from build123d import *

# Parameters (mm, degrees)
SKETCH1_W                                           = 162
SKETCH1_H                                           = 180
SKETCH1_W_2                                         = 50
SKETCH1_H_2                                         = 4
SKETCH1_W_3                                         = 4
SKETCH1_H_3                                         = 50
BOSS_EXTRUDE2_DEPTH                                 = 4
CUT_EXTRUDE1_REACH                                  = 136.376
SKETCH2_W                                           = 50
SKETCH2_H                                           = 4
CSK_FOR_M3_COUNTERSUNK_FLAT_HEAD_SCREW1_D           = 3.4
CSK_FOR_M3_COUNTERSUNK_FLAT_HEAD_SCREW1_CSINK_D     = 6.3
CSK_FOR_M3_COUNTERSUNK_FLAT_HEAD_SCREW1_CSINK_ANGLE = 90
CSK_FOR_M4_COUNTERSUNK_FLAT_HEAD_SCR_2_COUNT        = 2
CSK_FOR_M4_COUNTERSUNK_FLAT_HEAD_SCR_2_PITCH        = 142
CSK_FOR_M4_COUNTERSUNK_FLAT_HEAD_SCR_3_COUNT        = 2
CSK_FOR_M4_COUNTERSUNK_FLAT_HEAD_SCR_3_PITCH        = 205.104851235
CSK_FOR_M4_COUNTERSUNK_FLAT_HEAD_SCR_4_COUNT        = 2
CSK_FOR_M4_COUNTERSUNK_FLAT_HEAD_SCR_4_PITCH        = 148
CSK_FOR_M3_COUNTERSUNK_FLAT_HEAD_SCREW3_D           = 3.4
CSK_FOR_M3_COUNTERSUNK_FLAT_HEAD_SCREW3_CSINK_D     = 6.3
CSK_FOR_M3_COUNTERSUNK_FLAT_HEAD_SCREW3_CSINK_ANGLE = 90


with BuildPart() as part:
    # Sketch1 → Boss-Extrude2 (new body)
    with BuildSketch(Plane.XY):
        with Locations((0, 10)):
            Rectangle(SKETCH1_W, SKETCH1_H)
        with Locations((0, 102)):
            Rectangle(SKETCH1_W_2, SKETCH1_H_2)
        with Locations((83, 10)):
            Rectangle(SKETCH1_W_3, SKETCH1_H_3)
        with Locations((-83, 10)):
            Rectangle(SKETCH1_W_3, SKETCH1_H_3)
    extrude(amount=BOSS_EXTRUDE2_DEPTH)

    # Sketch2 → Cut-Extrude1 (cut, up to next)
    with BuildSketch(Plane.XY.offset(4), mode=Mode.PRIVATE) as cut_extrude1_sk1:
        with Locations((0, -70)):
            Rectangle(SKETCH2_W, SKETCH2_H)
    cut_extrude1_tool1 = extrude(cut_extrude1_sk1.sketch, amount=-CUT_EXTRUDE1_REACH, mode=Mode.PRIVATE) & part.part
    add(cut_extrude1_tool1.solids().sort_by_distance((0, -70, 4))[0], mode=Mode.SUBTRACT)

    # CSK for M3 Countersunk Flat Head Screw1 (through all)
    with Locations(Plane(origin=(-44, 54, 4), x_dir=(1, 0, 0), z_dir=(0, 0, 1))):
        with Locations((0, 0), (88, 0), (88, -38), (0, -38)):
            CounterSinkHole(CSK_FOR_M3_COUNTERSUNK_FLAT_HEAD_SCREW1_D / 2, CSK_FOR_M3_COUNTERSUNK_FLAT_HEAD_SCREW1_CSINK_D / 2, counter_sink_angle=CSK_FOR_M3_COUNTERSUNK_FLAT_HEAD_SCREW1_CSINK_ANGLE)

    # Sketch6 → CSK for M4 Countersunk Flat Head Screw1 (revolve, cut)
    with BuildSketch(Plane(origin=(-71, 90, 4), x_dir=(0, -1, 0), z_dir=(1, 0, 0))):
        Polygon((0, 0), (0, 4), (2.25, 4), (2.25, 2.45), (4.7, 0), align=None)
    csk_for_m4_countersunk_flat_head_screw1 = revolve(axis=Axis((-71, 90, 10.35), (0, 0, -1)), mode=Mode.SUBTRACT)

    # CSK for M4 Countersunk Flat Head Scr 2: CSK for M4 Countersunk Flat Head Screw1 ×2
    with Locations(*[(i * CSK_FOR_M4_COUNTERSUNK_FLAT_HEAD_SCR_2_PITCH, 0, 0) for i in range(1, CSK_FOR_M4_COUNTERSUNK_FLAT_HEAD_SCR_2_COUNT)]):
        add(csk_for_m4_countersunk_flat_head_screw1, mode=Mode.SUBTRACT)

    # CSK for M4 Countersunk Flat Head Scr 3: CSK for M4 Countersunk Flat Head Screw1 ×2
    with Locations(*[Vector(0.6923288217962463, -0.7215821522946791, 0) * (i * CSK_FOR_M4_COUNTERSUNK_FLAT_HEAD_SCR_3_PITCH) for i in range(1, CSK_FOR_M4_COUNTERSUNK_FLAT_HEAD_SCR_3_COUNT)]):
        add(csk_for_m4_countersunk_flat_head_screw1, mode=Mode.SUBTRACT)

    # CSK for M4 Countersunk Flat Head Scr 4: CSK for M4 Countersunk Flat Head Screw1 ×2
    with Locations(*[(0, -i * CSK_FOR_M4_COUNTERSUNK_FLAT_HEAD_SCR_4_PITCH, 0) for i in range(1, CSK_FOR_M4_COUNTERSUNK_FLAT_HEAD_SCR_4_COUNT)]):
        add(csk_for_m4_countersunk_flat_head_screw1, mode=Mode.SUBTRACT)

    # CSK for M3 Countersunk Flat Head Screw3 (through all)
    with Locations(Plane(origin=(-39, -10.5, 4), x_dir=(1, 0, 0), z_dir=(0, 0, 1))):
        with Locations((0, 0), (78, -47.5)):
            CounterSinkHole(CSK_FOR_M3_COUNTERSUNK_FLAT_HEAD_SCREW3_D / 2, CSK_FOR_M3_COUNTERSUNK_FLAT_HEAD_SCREW3_CSINK_D / 2, counter_sink_angle=CSK_FOR_M3_COUNTERSUNK_FLAT_HEAD_SCREW3_CSINK_ANGLE)


solid = part.part
Design review of the part built by this model. Coordinates are the model's own, in mm. A direction names the side the tool comes from. Coordinates: 2 decimals unless noted, no trailing zeros. Order: outer loops, then holes, each group sorted by start corner. A loop starts at its lowest first (then second) coordinate and runs counter-clockwise, first axis right, second up. Notation, with made-up numbers: M -13,-17.75 L 6,-17.75 A36 ccw 6,17.25 Z; hole C -4,-19 d5. An arc over 180 degrees is marked long. Use a Markdown table: item, result.
(1) Add section A-A (z = 0.65). Count the separate pieces of the cut face and the enclosed holes in it, then the cut area to 3 significant figures.
Worked answers:
| item | result |
|---|---|
| separate pieces | 1 |
| enclosed holes | 11 |
| area | 29,400 mm2 |
(2) For faces 1 (the flat face through (-81, -48, 2)), 2 (the flat face through (-53, 100, 2)), 3 (the flat face through (53, 100, 2)), list the 3-axis set-ups (+Z, -Z, +X, -X, +Y, -Y) from which the entire face can be reached by the end or side of a thin tool; tool diameter is ignored.
Worked answers:
| item | result |
|---|---|
| face 1 | +Z, -Z, -X, -Y |
| face 2 | +Z, -Z, -X, +Y |
| face 3 | +Z, -Z, +X, +Y |
(3) Add section B-B (y = 90). Give the boundary of the cut face in (x, z).
Worked answers:
| item | result |
|---|---|
| outline | M -81,0 L -73.25,0 L -73.25,1.55 L -75.7,4 L -81,4 Z; M -68.75,0 L 68.75,0 L 68.75,1.55 L 66.3,4 L -66.3,4 L -68.75,1.55 Z; M 73.25,0 L 81,0 L 81,4 L 75.7,4 L 73.25,1.55 Z |
(4) For P1, Ø2, axis at y = 52.5, z = 2, coming from the +X side; P2, Ø1.2, axis at x = -83, z = 2.5, coming from the +Y side; P3, Ø5, axis at x = -71, y = 90, coming from the +Z side, all flat-tipped, find the tip position at first contact; note any pin that passes through.
Worked answers:
| item | result |
|---|---|
| P1 | stops at x = 81 |
| P2 | stops at y = 35 |
| P3 | stops at z = 1.8 |
(5) Wall thickness on probe 1 along X at (y, z) = (16, 1.25); probe 2 along Y at (x, z) = (-44, 1.7); probe 3 along Y at (x, z) = (14, 3.45): over which ranges is each line inside the solid? List them lowest first.
Worked answers:
| item | result |
|---|---|
| probe 1 | x = -85 to -45.7, -42.3 to 42.3, 45.7 to 85 |
| probe 2 | y = -80 to 14.3, 17.7 to 52.3, 55.7 to 100 |
| probe 3 | y = -80 to -72, -68 to 104 |
(6) Draft analysis for pull direction Y (two halves, no side actions). For faces 4 (the flat face through (-83, 35, 2)), 5 (the cylindrical face through (71.86, 87.92, 0.79)), 6 (the flat face through (-83, -15, 2)), 7 (the cylindrical face through (-68.804, -57.512, 0.786)), state which applies: released by +Y, released by -Y, zero draft, split by the parting line, or undercut.
Worked answers:
| item | result |
|---|---|
| face 4 | released by +Y |
| face 5 | undercut |
| face 6 | released by -Y |
| face 7 | undercut |
(7) Add section D-D (y = -36.5). Give the boundary of the cut face in (x, z).
Worked answers:
| item | result |
|---|---|
| outline | M -81,0 L 81,0 L 81,4 L -81,4 Z |
(8) Add section C-C (x = -62.5). Give the boundary of the cut face in (y, z).
Worked answers:
| item | result |
|---|---|
| outline | M -80,0 L 100,0 L 100,4 L -80,4 Z |
